from build123d import *

# Parameters (mm, degrees)
SKETCH1_R           = 9.75
BOSS_EXTRUDE1_DEPTH = 3.175


with BuildPart() as part:
    # Sketch1 → Boss-Extrude1 (new body)
    with BuildSketch(Plane.XY.offset(3.175)):
        Circle(SKETCH1_R)
        Polygon((-3.739497694, 6.477), (3.739497694, 6.477), (7.478995387, 0), (3.739497694, -6.477), (-3.739497694, -6.477), (-7.478995387, 0), align=None, mode=Mode.SUBTRACT)
    extrude(amount=-BOSS_EXTRUDE1_DEPTH)


solid = part.part
Geometry check sheet. Reference: the model listing, model coordinates, mm. A direction names the side the tool comes from. Coordinates: 2 decimals unless noted, no trailing zeros. Order: outer loops, then holes, each group sorted by start corner. A loop starts at its lowest first (then second) coordinate and runs counter-clockwise, first axis right, second up. Notation, with made-up numbers: (-5, 4.5) - (1, 4.5) arc R4 ccw to (1, 9.5) - close; hole circle Ø2 at (26.5, 3.25). An arc over 180 degrees is marked (long way). Answer in a Markdown table with one row per item. Add a question column.
1) Cross-section at C-C, the plane y = 1.25. Record the cut outline in (x, z) (3 decimals).
2) Cross-section at B-B, the plane z = 2.5. Record the cut outline in (x, y), then the cut area to 3 significant figures.
3) Cross-section at A-A, the plane x = 0. Record the cut outline in (y, z) (3 decimals), then the cut area to 3 significant figures.
4) Material ranges on line 1 along Y through (x, z) = (0.25, 0.65); line 2 along Y through (x, z) = (-4.25, 2); line 3 along X through (y, z) = (4.25, 2.5), recorded low to high. Write a range as [from, to].
5) Set-up check for faces 1 (the flat face through (6.4, 2.3, 0)), 2 (the flat face through (0, -6.477, 2)): record each of +Z, -Z, +X, -X, +Y, -Y from which the full face is reachable in a straight line by a thin tool's end or side.
6) Cross-section at D-D, the plane y = 7.25. Record the cut outline in (x, z) (3 decimals).
7) Release check for a two-part mould opening along X. For faces 3 (the flat face through (-5.635, 3.193, 1.61)), 4 (the cylindrical face through (-1.269, 9.667, 1.61)), 5 (the flat face through (6.4, 2.3, 3.175)), 6 (the flat face through (-5.583, -3.284, 1.61)) record: +X half, -X half, draft (parallel to the pull), parting line (faces both ways), or undercut.
Check result:
| question | item | result |
|---|---|---|
| 1 | outline | (-9.67, 0) - (-6.757, 0) - (-6.757, 3.175) - (-9.67, 3.175) - close; (6.757, 0) - (9.67, 0) - (9.67, 3.175) - (6.757, 3.175) - close |
| 2 | outline | circle Ø19.5 at (0, 0); hole (-7.48, 0) - (-3.74, -6.48) - (3.74, -6.48) - (7.48, 0) - (3.74, 6.48) - (-3.74, 6.48) - close |
| 2 | area | 153 mm² |
| 3 | outline | (-9.75, 0) - (-6.477, 0) - (-6.477, 3.175) - (-9.75, 3.175) - close; (6.477, 0) - (9.75, 0) - (9.75, 3.175) - (6.477, 3.175) - close |
| 3 | area | 20.8 mm² |
| 4 | line 1 | y = [-9.75, -6.48], [6.48, 9.75] |
| 4 | line 2 | y = [-8.77, -5.59], [5.59, 8.77] |
| 4 | line 3 | x = [-8.77, -5.03], [5.03, 8.77] |
| 5 | face 1 | -Z, +X, -X, +Y, -Y |
| 5 | face 2 | +Z, -Z |
| 6 | outline | (-6.519, 0) - (6.519, 0) - (6.519, 3.175) - (-6.519, 3.175) - close |
| 7 | face 3 | undercut |
| 7 | face 4 | parting line |
| 7 | face 5 | draft |
| 7 | face 6 | undercut |
